Part model, mm, in its own coordinate system. Face numbers are marked on the shaded views. A direction names the side the tool comes from. Give positions to 0.01 mm unless a question says otherwise; leave off trailing zeros. Write each loop counter-clockwise with the first axis right and the second up, starting at its lowest first coordinate (ties: lowest second). Pieces come first, ordered by that corner, then holes. Notation, with made-up numbers: M -14.5,68.5 L 33.5,68.5 A25 cw 33.5,88.5 Z; hole C 34.5,83 d6. An arc over 180 degrees is marked long. Answer as CSV lines item,"result". Start each with the question number.
1) Slice it at A-A, the plane y = 19. Give the cut face in (x, z), plus the area to 3 significant figures.
2) Mould opens along Y. For the marked faces 4, 5 and 6 say: pulls with the +Y half, pulls with the -Y half, needs draft (parallel to the pull), parting line crosses it, or undercut.
3) Slice it at C-C, the plane z = -3. Give the cut face in (x, y), plus the area to 3 significant figures.
4) Tool access for the marked faces 1, 2 and 3: list every direction of +Z, -Z, +X, -X, +Y, -Y with a clear straight run to the whole face (end or side of a thin tool).
5) Slice it at D-D, the plane z = 5. Give the cut face in (x, y), plus the area to 3 significant figures.
6) Wall check: line 1 along Z through (x, y) = (-4, 28); line 2 along Y through (x, z) = (28, 1); line 3 along X through (y, z) = (35, -6.5). Give the ranges that are in metal, low to high. Write a range as from..to.
7) Slice it at B-B, the plane x = 4. Give the cut face in (y, z).
8) Pin check, flat tips, straight feed: pin 1 Ø5 at (y, z) = (26.5, -10) entering from +X; pin 2 Ø8.5 at (x, z) = (-3, 4.5) entering from +Y; pin 3 Ø1 at (x, y) = (-2, 33) entering from -Z. Stop position of each tip, or through.
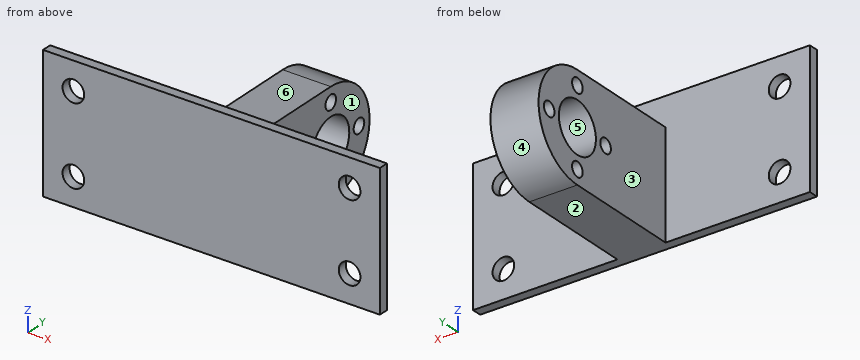
```python
from build123d import *

# Parameters (mm, degrees)
SKETCH1_W                = 70
SKETCH1_H                = 28
BOSS_EXTRUDE1_DEPTH      = 2
SKETCH2_R                = 11
SKETCH2_R_2              = 5.25
BOSS_EXTRUDE2_DEPTH      = 5
BOSS_EXTRUDE3_REACH      = 54.125
BOSS_EXTRUDE3_END_RADIUS = 11
SKETCH3_W                = 10
SKETCH3_H                = 22
SKETCH5_R                = 2.25
CUT_EXTRUDE1_DEPTH       = 53.12485012
MIRROR2_COPY_1_SKETCH_R  = 2.25
MIRROR2_COPY_1_DEPTH     = 53.12485012
SKETCH6_R                = 1.5
CUT_EXTRUDE2_DEPTH       = 57.920997883


with BuildPart() as part:
    # Sketch1 → Boss-Extrude1 (new body)
    with BuildSketch(Plane(origin=(0, 0, 0), x_dir=(1, 0, 0), z_dir=(0, 1, 0))):
        Rectangle(SKETCH1_W, SKETCH1_H)
    extrude(amount=BOSS_EXTRUDE1_DEPTH)



with BuildPart() as body_2:
    # Sketch2 → Boss-Extrude2 (new, symmetric)
    with BuildSketch(Plane(origin=(0, 0, 0), x_dir=(0, 0, -1), z_dir=(1, 0, 0))):
        with Locations((3, 27)):
            Circle(SKETCH2_R)
        with Locations((3, 27)):
            Circle(SKETCH2_R_2, mode=Mode.SUBTRACT)
    extrude(amount=BOSS_EXTRUDE2_DEPTH, both=True)


with BuildPart() as part_1:
    add(part.part)

    add(body_2.part)  # Boss-Extrude3 merges body 2
    # Boss-Extrude3: up to this cylinder (the profile starts outside it)
    boss_extrude3_end = Plane(origin=(0, 27, -3), z_dir=(-1, 0, 0)) * Cylinder(BOSS_EXTRUDE3_END_RADIUS, 131.25, mode=Mode.PRIVATE)
    # Sketch3 → Boss-Extrude3 (add, up to the surface)
    with BuildSketch(Plane(origin=(0, 2, 0), x_dir=(1, 0, 0), z_dir=(0, 1, 0)), mode=Mode.PRIVATE) as boss_extrude3_sk1:
        with Locations((0, 3)):
            Rectangle(SKETCH3_W, SKETCH3_H)
    boss_extrude3_tool1 = extrude(boss_extrude3_sk1.sketch, amount=BOSS_EXTRUDE3_REACH, mode=Mode.PRIVATE) - boss_extrude3_end
    add(boss_extrude3_tool1.solids().sort_by_distance((0, 2, -3))[0])

    # Sketch5 → Cut-Extrude1 (cut, through all)
    with BuildSketch(Plane(origin=(0, 2, 0), x_dir=(1, 0, 0), z_dir=(0, 1, 0))):
        with Locations(Location((-28.692400687, 8.162233715, 0), (0, 0, 270))):
            Circle(SKETCH5_R)
    cut_extrude1 = extrude(amount=-CUT_EXTRUDE1_DEPTH, mode=Mode.SUBTRACT)

    # Mirror1: Cut-Extrude1 across plane
    add(cut_extrude1.mirror(Plane(origin=(0, 0, 0), x_dir=(1, 0, 0), z_dir=(0, 0, -1))), mode=Mode.SUBTRACT)

    # Mirror2: Cut-Extrude1 across plane
    add(cut_extrude1.mirror(Plane.ZY), mode=Mode.SUBTRACT)

    # Mirror2 copy 1 sketch → Mirror2 copy 1 (cut, through all)
    with BuildSketch(Plane(origin=(0, 2, 0), x_dir=(-1, 0, 0), z_dir=(0, 1, 0))):
        with Locations(Location((-28.692400687, 8.162233715, 0), (0, 0, 270))):
            Circle(MIRROR2_COPY_1_SKETCH_R)
    extrude(amount=-MIRROR2_COPY_1_DEPTH, mode=Mode.SUBTRACT)

    # Sketch6 → Cut-Extrude2 (cut, through all)
    with BuildSketch(Plane.ZY.offset(5)):
        with Locations((-3, 35)):
            Circle(SKETCH6_R)
        with Locations((-11, 27)):
            Circle(SKETCH6_R)
        with Locations((5, 27)):
            Circle(SKETCH6_R)
        with Locations((-3, 19)):
            Circle(SKETCH6_R)
    extrude(amount=-CUT_EXTRUDE2_DEPTH, mode=Mode.SUBTRACT)


solid = part_1.part
```
Found:
1,outline,"M -5,-14 L 5,-14 L 5,-4.5 L -5,-4.5 Z; M -5,-1.5 L 5,-1.5 L 5,8 L -5,8 Z"
1,area,"190 mm²"
2,face 4,"pulls with the +Y half"
2,face 5,"undercut"
2,face 6,"needs draft"
3,outline,"M -35,0 L 35,0 L 35,2 L 5,2 L 5,17.5 L -5,17.5 L -5,2 L -35,2 Z; M -5,20.5 L 5,20.5 L 5,21.75 L -5,21.75 Z; M -5,32.25 L 5,32.25 L 5,33.5 L -5,33.5 Z; M -5,36.5 L 5,36.5 L 5,38 L -5,38 Z"
3,area,"335 mm²"
4,face 1,"+Z, -Z, +X, +Y"
4,face 2,"-Z, +X, -X, +Y, -Y"
4,face 3,"+Z, -Z, -X, +Y"
5,outline,"M -35,0 L 35,0 L 35,2 L 5,2 L 5,25.5 L -5,25.5 L -5,2 L -35,2 Z; M -5,28.5 L 5,28.5 L 5,34.55 L -5,34.55 Z"
5,area,"435 mm²"
6,line 1,"-13.95..-12.12, -9.88..-8.15, 2.15..3.88, 6.12..7.95"
6,line 2,"0..2"
6,line 3,"-5..5"
7,outline,"M 0,-14 L 27,-14 A11 ccw 27,8 L 2,8 L 2,14 L 0,14 Z; hole C 19,-3 d3; hole C 27,-3 d10.5; hole C 27,-11 d3; hole C 27,5 d3; hole C 35,-3 d3"
8,pin 1,"x = 5"
8,pin 2,"y = 37.51"
8,pin 3,"z = -12.53"
